Here's the drawing with two shaded views (mm, measured from the low corner). I have some questions. Round coordinates to 2 decimals unless told otherwise and drop trailing zeros. Order: outer loops, then holes, each group sorted by start corner. A loop starts at its lowest first (then second) coordinate and runs counter-clockwise, first axis right, second up. Notation, with made-up numbers: (-9, -30.75) - (29, -30.75) arc R24 cw to (29, -6.75) - close; hole circle Ø1 at (71.5, 69.25). An arc over 180 degrees is marked (long way). One line per item, written item: value.
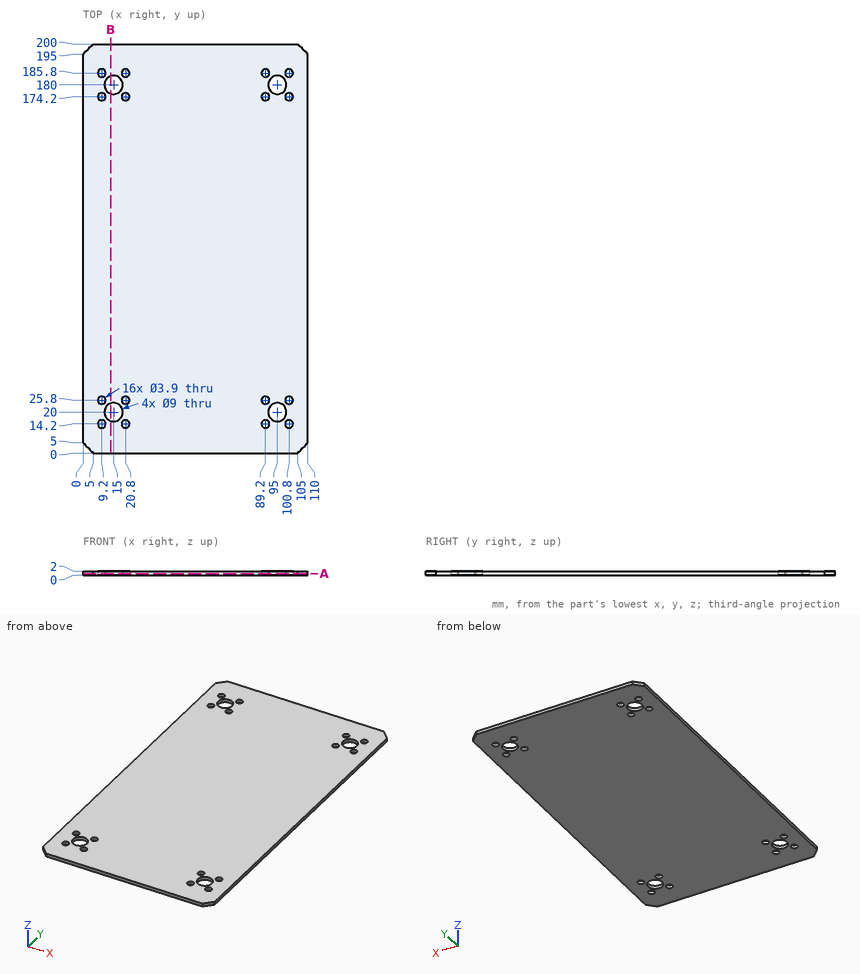
Q1. If we section it at A-A, the plane z = 0.75: Give the number of separate pieces and of enclosed holes in the cut face, then the cut area to 3 significant figures.
Results list:
separate pieces: 1
enclosed holes: 20
area: 21,500 mm²
Q2. If we section it at B-B, the plane x = 13.5: Please give me the cut outline in (y, z), then the cut area to 3 significant figures.
Results list:
outline: (0, 0) - (15.76, 0) - (15.76, 2) - (0, 2) - close; (24.24, 0) - (175.76, 0) - (175.76, 2) - (24.24, 2) - close; (184.24, 0) - (200, 0) - (200, 2) - (184.24, 2) - close
area: 366 mm²
Q3. Will these pins go through, and if not, where does the flat tip stop? pin 1 (3 mm diameter, centred on x = 20.8, y = 185.8, fed in from +Z); pin 2 (5 mm diameter, centred on x = 27, y = 95, fed in from -Z).
Results list:
pin 1: through
pin 2: z = 0
Q4. If I drill on line 1 along Y through (x, z) = (15, 1.5); line 2 along Y through (x, z) = (100.8, 0.8); line 3 along X through (y, z) = (179.5, 0.65), over which ranges is the centre line in solid material (lowest first)?
Results list:
line 1: 0 to 15.5, 24.5 to 175.5, 184.5 to 200
line 2: 0 to 12.25, 16.15 to 23.85, 27.75 to 172.25, 176.15 to 183.85, 187.75 to 200
line 3: 0 to 10.53, 19.47 to 90.53, 99.47 to 110
